Read the model definition and answer for the solid it produces. Units are mm, in the model's axes. Face numbers are marked on the shaded views. A direction names the side the tool comes from. Round coordinates to 2 decimals unless told otherwise and drop trailing zeros. Order: outer loops, then holes, each group sorted by start corner. A loop starts at its lowest first (then second) coordinate and runs counter-clockwise, first axis right, second up. Notation, with made-up numbers: (81, 59.25) - (86, 59.25) arc R17 ccw to (86, 78.25) - close; hole circle Ø5 at (63.25, -17). An arc over 180 degrees is marked (long way). One line per question, with ' | ' between items. Start each with the question number.
1) The part is cut by section B-B, the plane z = 69. Give the vertices of the cut face in (x, y).
2) The part is cut by section C-C, the plane x = 12.25. Give the vertices of the cut face in (y, z), plus the area to 3 significant figures.
3) Straight lines are drawn through the part: line 1 (Z direction, x = 16.5, y = 3); line 2 (Y direction, x = 5.25, z = 12); line 3 (Y direction, x = 19.5, z = 38.5). For each, find the intervals that lie inside material, in ascending order. Write a range as from..to.
4) For the marked faces 1 and 2, determine the directions among +Z, -Z, +X, -X, +Y, -Y from which every point of the face is accessible in a straight line to the end or side of a thin tool.
5) The mould has two halves that part along Z. Classify the marked faces 3, 4 and 5: pulls with the +Z half, pulls with the -Z half, needs draft (parallel to the pull), parting line crosses it, or undercut.
6) The part is cut by section A-A, the plane y = 2.5. Give the vertices of the cut face in (x, z), plus the area to 3 significant figures.
7) A flat-ended cylindrical pin translates along its axis: pin 1 (3 mm diameter, centred on x = 22, z = 31.5, fed in from -Y). Find the tip coordinate at first contact, or state that the pin passes through.
8) The part is cut by section D-D, the plane z = 14. Give the vertices of the cut face in (x, y), plus the area to 3 significant figures.
from build123d import *

# Parameters (mm, degrees)
F0_W         = 25
F0_H         = 20
F1_DEPTH     = 93
F3_R         = 80
F3_R_2       = 65
F4_DEPTH     = 30
F6_T1_DEPTH  = 10
F6_T3_DEPTH  = 15
F6_T5_DEPTH  = 100.5
F6_S9_W      = 5
F6_S9_H      = 5
F6_T10_DEPTH = 5
F6_S15_W     = 5
F6_S15_H     = 5
F6_T16_DEPTH = 5
F6_S21_W     = 5
F6_S21_H     = 5
F6_T22_DEPTH = 5
F6_S27_W     = 5
F6_S27_H     = 5
F6_T28_DEPTH = 5


# Not quite as in the source:
# - a fillet or chamfer that OpenCascade refuses, or shapes differently, is made with other operations: its cross-section is extruded or revolved along the edge and cut away or added


with BuildPart() as f1:
    # F0 (on Top) → F1 (new body)
    with BuildSketch(Plane.XY):
        with Locations((12.5, 0)):
            Rectangle(F0_W, F0_H)
    extrude(amount=F1_DEPTH)


with BuildPart() as f4:
    # F3 (on offset) → F4 (new body)
    with BuildSketch(Plane.XY.offset(10)):
        with Locations((10.065856821, 72.5)):
            Circle(F3_R)
        with Locations((10.065856821, 72.5)):
            Circle(F3_R_2, mode=Mode.SUBTRACT)
    extrude(amount=F4_DEPTH)


with BuildPart() as f1_1:
    add(f1.part)

    # F5: cut F4
    add(f4.part, mode=Mode.SUBTRACT)

    # F6: fillet of radius 5 on 8 edges, made by hand

    # F6_s2 → F6_t1 (cut)
    with BuildSketch(Plane.XZ.offset(-5)):
        with BuildLine():
            ThreePointArc((0, 5), (1.4644660941, 1.4644660941), (5, 0))
            Line((5, 0), (0, 0))
            Line((0, 0), (0, 5))
        make_face()
        with BuildLine():
            ThreePointArc((25, 5), (23.5355339059, 1.4644660941), (20, 0))
            Line((20, 0), (25, 0))
            Line((25, 0), (25, 5))
        make_face()
    extrude(amount=F6_T1_DEPTH, mode=Mode.SUBTRACT)

    # F6_s4 → F6_t3 (cut)
    with BuildSketch(Plane.YZ.offset(5)):
        with BuildLine():
            ThreePointArc((10, 5), (8.5355339059, 1.4644660941), (5, 0))
            Line((5, 0), (10, 0))
            Line((10, 0), (10, 5))
        make_face()
        with BuildLine():
            ThreePointArc((-5, 0), (-8.5355339059, 1.4644660941), (-10, 5))
            Line((-10, 5), (-10, 0))
            Line((-10, 0), (-5, 0))
        make_face()
    extrude(amount=F6_T3_DEPTH, mode=Mode.SUBTRACT)

    # F6_s6 → F6_t5 (cut)
    with BuildSketch(Plane.XY.offset(5)):
        with BuildLine():
            ThreePointArc((25, -5), (23.5355339059, -8.5355339059), (20, -10))
            Line((20, -10), (25, -10))
            Line((25, -10), (25, -5))
        make_face()
        with BuildLine():
            ThreePointArc((0, -5), (1.4644660941, -8.5355339059), (5, -10))
            Line((5, -10), (0, -10))
            Line((0, -10), (0, -5))
        make_face()
        with BuildLine():
            ThreePointArc((5, 10), (1.4644660941, 8.5355339059), (0, 5))
            Line((0, 5), (0, 10))
            Line((0, 10), (5, 10))
        make_face()
        with BuildLine():
            ThreePointArc((20, 10), (23.5355339059, 8.5355339059), (25, 5))
            Line((25, 5), (25, 10))
            Line((25, 10), (20, 10))
        make_face()
    extrude(amount=F6_T5_DEPTH, mode=Mode.SUBTRACT)


with BuildPart() as f6_tool8:
    # F6_s9 → F6_t10 (new body)
    with BuildSketch(Plane.XZ.offset(-5)):
        with Locations((2.5, 2.5)):
            Rectangle(F6_S9_W, F6_S9_H)
    extrude(amount=-F6_T10_DEPTH)

    # F6_s11 → F6_t12 (revolve, cut)
    with BuildSketch(Plane(origin=(5, 5, 5), x_dir=(0.7071067812, 0, 0.7071067812), z_dir=(-0.7071067812, 0, 0.7071067812))):
        with BuildLine():
            ThreePointArc((0, -5), (5, 0), (0, 5))
            Line((0, 5), (0, -5))
        make_face()
    revolve(axis=Axis((5, 5, 5), (0, 1, 0)), mode=Mode.SUBTRACT)


with BuildPart() as f1_2:
    add(f1_1.part)

    # F6_t7: cut F6_tool8
    add(f6_tool8.part, mode=Mode.SUBTRACT)


with BuildPart() as f6_tool14:
    # F6_s15 → F6_t16 (new body)
    with BuildSketch(Plane.YZ.offset(5)):
        with Locations((-7.5, 2.5)):
            Rectangle(F6_S15_W, F6_S15_H)
    extrude(amount=-F6_T16_DEPTH)

    # F6_s17 → F6_t18 (revolve, cut)
    with BuildSketch(Plane(origin=(5, -5, 5), x_dir=(0, 0.7071067812, 0.7071067812), z_dir=(0, -0.7071067812, 0.7071067812))):
        with BuildLine():
            ThreePointArc((0, -5), (5, 0), (0, 5))
            Line((0, 5), (0, -5))
        make_face()
    revolve(axis=Axis((5, -5, 5), (-1, 0, 0)), mode=Mode.SUBTRACT)


with BuildPart() as f1_3:
    add(f1_2.part)

    # F6_t13: cut F6_tool14
    add(f6_tool14.part, mode=Mode.SUBTRACT)


with BuildPart() as f6_tool20:
    # F6_s21 → F6_t22 (new body)
    with BuildSketch(Plane.XZ.offset(-5)):
        with Locations((22.5, 2.5)):
            Rectangle(F6_S21_W, F6_S21_H)
    extrude(amount=-F6_T22_DEPTH)

    # F6_s23 → F6_t24 (revolve, cut)
    with BuildSketch(Plane(origin=(20, 5, 5), x_dir=(-0.7071067812, 0, 0.7071067812), z_dir=(-0.7071067812, 0, -0.7071067812))):
        with BuildLine():
            ThreePointArc((0, -5), (5, 0), (0, 5))
            Line((0, 5), (0, -5))
        make_face()
    revolve(axis=Axis((20, 5, 5), (0, 1, 0)), mode=Mode.SUBTRACT)


with BuildPart() as f1_4:
    add(f1_3.part)

    # F6_t19: cut F6_tool20
    add(f6_tool20.part, mode=Mode.SUBTRACT)


with BuildPart() as f6_tool26:
    # F6_s27 → F6_t28 (new body)
    with BuildSketch(Plane.YZ.offset(20)):
        with Locations((-7.5, 2.5)):
            Rectangle(F6_S27_W, F6_S27_H)
    extrude(amount=F6_T28_DEPTH)

    # F6_s29 → F6_t30 (revolve, cut)
    with BuildSketch(Plane(origin=(20, -5, 5), x_dir=(0, 0.7071067812, 0.7071067812), z_dir=(0, 0.7071067812, -0.7071067812))):
        with BuildLine():
            ThreePointArc((0, -5), (5, 0), (0, 5))
            Line((0, 5), (0, -5))
        make_face()
    revolve(axis=Axis((20, -5, 5), (1, 0, 0)), mode=Mode.SUBTRACT)


with BuildPart() as f1_5:
    add(f1_4.part)

    # F6_t25: cut F6_tool26
    add(f6_tool26.part, mode=Mode.SUBTRACT)


solid = f1_5.part
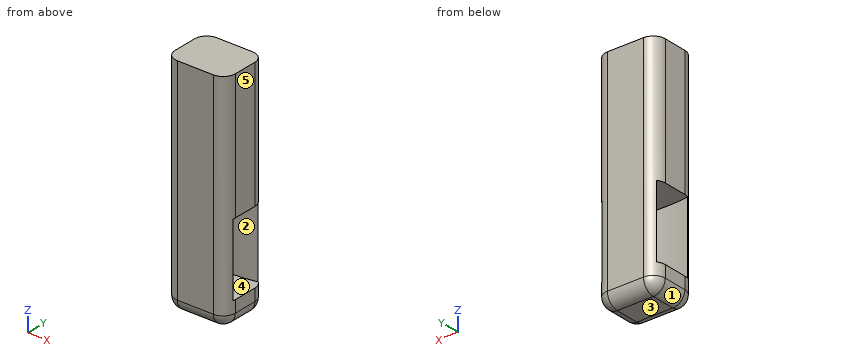
Values:
1) outline: (0, -5) arc R5 ccw to (5, -10) - (20, -10) arc R5 ccw to (25, -5) - (25, 5) arc R5 ccw to (20, 10) - (5, 10) arc R5 ccw to (0, 5) - close
2) outline: (-10, 5) arc R5 ccw to (-5, 0) - (5, 0) arc R5 ccw to (10, 5) - (10, 93) - (-10, 93) - close; hole (-7.47, 10) - (7.54, 10) - (7.54, 40) - (-7.47, 40) - close | area: 1,400 mm^2
3) line 1: z = 0..10, 40..93 | line 2: y = -10..-7.35, 7.68..10 | line 3: y = -10..-6.94, 8.19..10
4) face 1: -Z, -X, +Y, -Y | face 2: none
5) face 3: pulls with the -Z half | face 4: undercut | face 5: needs draft
6) outline: (0, 5) arc R5 ccw to (5, 0) - (20, 0) arc R5 ccw to (25, 5) - (25, 10) - (0, 10) - close; (0, 40) - (25, 40) - (25, 93) - (0, 93) - close | area: 1,560 mm^2
7) pin 1: stops at y = -9.97
8) outline: (0.38, -6.91) arc R5 ccw to (5, -10) - (20, -10) arc R5 ccw to (24.87, -6.12) arc R80 cw to start; (1.09, 8.12) arc R65 ccw to (23.2, 8.84) arc R5 ccw to (20, 10) - (5, 10) arc R5 ccw to start | area: 105 mm^2
